Autodesk Inventor part; units mm, degrees
ref_plane "YZ Plane" through (0, 0, 0) normal (1, 0, 0) x (0, 1, 0)
ref_plane "XZ Plane" through (0, 0, 0) normal (0, 1, 0) x (-1, 0, 0)
ref_plane "XY Plane" through (0, 0, 0) normal (0, 0, 1) x (1, 0, 0)
sketch "Boceto1" plane through (0, 0, 0) normal (0, 1, 0) x (-1, 0, 0)
  line L0 (70.0475, 27.7623) -> (-31.8125, 27.7623)
  line L1 (-31.8125, 27.7623) -> (-31.8125, -25.8477)
  line L2 (-31.8125, -25.8477) -> (70.0475, -25.8477)
  line L3 (70.0475, -25.8477) -> (70.0475, 27.7623)
  point P0 (0, 0)
  dimension "d0" = 53.61
  dimension "d1" = 101.86
extrude "Extrusión1" add sketch "Boceto1" along normal blind 2
sketch "Boceto6" plane through (0, 0, 0) normal (0, -1, 0) x (1, 0, 0)
  line L0 (-50.0475, 27.7623) -> (23.8125, 27.7623)
  line L1 (28.8125, 27.7623) -> (31.8125, 24.7623)
  line L2 (31.8125, 27.7623) -> (31.8125, -25.8477)
  line L3 (-70.0475, 27.7623) -> (31.8125, 27.7623)
  line L4 (28.8125, 27.7623) -> (31.8125, 27.7623)
  line L5 (31.8125, 27.7623) -> (31.8125, 24.7623)
  circle A0 centre (25.3125, 25.7623) radius 1.5
  line L6 (31.8125, 17.7623) -> (31.8125, -25.8477)
  line L7 (31.8125, -15.8477) -> (25.8125, -25.8477)
  line L8 (31.8125, -25.8477) -> (23.8125, -25.8477)
  line L9 (31.8125, -25.8477) -> (28.8125, -25.8477)
  line L10 (28.8125, -25.8477) -> (28.8125, 5.0493)
  line L11 (28.8125, -10.8477) -> (31.8125, -5.8477)
  line L12 (31.8125, -5.8477) -> (31.8125, -25.8477)
  line L13 (25.8125, -25.8477) -> (31.8125, -25.8477)
  circle A1 centre (16.8125, -23.8477) radius 1.5
  line L14 (31.8125, -25.8477) -> (-70.0475, -25.8477)
  circle A2 centre (-56.0475, 25.7623) radius 1.5
  line L15 (-70.0475, 27.7623) -> (31.8125, 27.7623)
  line L16 (-70.0475, -25.8477) -> (-70.0475, 27.7623)
  circle A3 centre (-55.0475, -23.8477) radius 1.5
  point P0 (0, 0)
  point P1 (28.8125, -20.8477)
  point P2 (28.8125, -20.8477)
  dimension "d39" = 3
  dimension "d40" = 3
  dimension "d41" = 3
  dimension "d42" = 6.5
  dimension "d43" = 2
  dimension "d44" = 6
  dimension "d45" = 10
  dimension "d46" = 3
  dimension "d47" = 10
  dimension "d48" = 10
  dimension "d49" = 3
  dimension "d50" = 2
  dimension "d51" = 15
  dimension "d52" = 3
  dimension "d53" = 2
  dimension "d54" = 14
  dimension "d55" = 3
  dimension "d56" = 2
  dimension "d57" = 15
extrude "Extrusión7" cut sketch "Boceto6" against normal blind 3 contours L3 L2 L1 | L7 L10 L8 | L2 L7 L10 L11 | L7 L2 L8 L10 | A0 | A1 | A2 | A3
sketch "Boceto5" plane through (0, 2, 0) normal (0, 1, 0) x (1, 0, 0)
  line L0 (-73.0475, -22.7623) -> (-58.0475, -22.7623)
  line L1 (-58.0475, -22.7623) -> (-58.0475, -15.7623)
  line L2 (-58.0475, -15.7623) -> (-73.0475, -15.7623)
  line L3 (-73.0475, -15.7623) -> (-73.0475, -22.7623)
  line L4 (-70.0475, -27.7623) -> (31.8125, -27.7623)
  line L5 (-70.0475, 25.8477) -> (-70.0475, -27.7623)
  point P0 (0, 0)
  point P1 (-50.0475, -27.7623)
  point P2 (-65.5475, -22.7623)
  dimension "d33" = 5
  dimension "d34" = 7
  dimension "d35" = 3
  dimension "d36" = 15
extrude "Extrusión6" add sketch "Boceto5" along normal blind 8
sketch "Boceto4" plane through (0, 2, 0) normal (0, 1, 0) x (1, 0, 0)
  line L0 (-52.9032, 4.2581) -> (-20.9032, 4.2581)
  line L1 (-20.9032, 4.2581) -> (-20.9032, 9.2581)
  line L2 (-20.9032, 9.2581) -> (-52.9032, 9.2581)
  line L3 (-52.9032, 9.2581) -> (-52.9032, 4.2581)
  line L4 (-1.1875, -7.7419) -> (3.8125, -7.7419)
  line L5 (3.8125, -7.7419) -> (3.8125, 4.2581)
  line L6 (3.8125, 4.2581) -> (-1.1875, 4.2581)
  line L7 (-1.1875, 4.2581) -> (-1.1875, -7.7419)
  line L8 (23.8125, 25.8477) -> (23.8125, -17.7623)
  point P0 (0, 0)
  point P1 (-36.9032, 9.2581)
  point P2 (-36.9032, 4.2581)
  point P3 (1.3125, 4.2581)
  point P4 (1.3125, -7.7419)
  point P5 (-1.1875, -1.7419)
  point P6 (3.8125, -1.7419)
  point P7 (-20.9032, 6.7581)
  point P8 (-52.9032, 6.7581)
  dimension "d19" = 5
  dimension "d20" = 12
  dimension "d21" = 5
  dimension "d22" = 32
  dimension "d23" = 20
extrude "Extrusión4" add sketch "Boceto4" along normal blind 8
sketch "Boceto7" plane through (0, 2, 0) normal (0, 1, 0) x (1, 0, 0)
  line L0 (27.3125, 20.8477) -> (22.3125, 20.8477)
  line L1 (22.3125, 20.8477) -> (22.3125, -22.1523)
  line L2 (22.3125, -22.1523) -> (27.3125, -22.1523)
  line L3 (27.3125, -22.1523) -> (27.3125, 20.8477)
  line L4 (28.8125, 10.8477) -> (28.8125, 20.8477)
  line L5 (25.8125, 25.8477) -> (-70.0475, 25.8477)
  line L6 (21.8125, -23.2623) -> (-43.1875, -23.2623)
  line L7 (-43.1875, -23.2623) -> (-43.1875, -26.2623)
  line L8 (-43.1875, -26.2623) -> (21.8125, -26.2623)
  line L9 (21.8125, -26.2623) -> (21.8125, -23.2623)
  line L10 (-70.0475, -27.7623) -> (28.8125, -27.7623)
  line L11 (31.8125, -24.7623) -> (31.8125, 5.8477)
  line L12 (13.8125, 24.3477) -> (-52.0475, 24.3477)
  line L13 (-52.0475, 24.3477) -> (-52.0475, 21.3477)
  line L14 (-52.0475, 21.3477) -> (13.8125, 21.3477)
  line L15 (13.8125, 21.3477) -> (13.8125, 24.3477)
  line L16 (-70.0475, 25.8477) -> (-70.0475, -15.7623)
  point P0 (0, 0)
  point P1 (24.8125, 20.8477)
  point P2 (21.8125, -24.7623)
  point P3 (-43.1875, -24.7623)
  point P4 (13.8125, 22.8477)
  point P5 (-52.0475, 22.8477)
  dimension "d60" = 1.5
  dimension "d61" = 5
  dimension "d62" = 5
  dimension "d63" = 43
  dimension "d64" = 1.5
  dimension "d65" = 3
  dimension "d66" = 10
  dimension "d67" = 65
  dimension "d68" = 1.5
  dimension "d69" = 3
  dimension "d70" = 15
  dimension "d71" = 18
extrude "Extrusión8" add sketch "Boceto7" along normal blind 8
properties part number "Wemos Mega"
Here's how the part is built. I have some questions about the finished solid (model axes, mm). A direction names the side the tool comes from. Coordinates: 2 decimals unless noted, no trailing zeros. Loops run counter-clockwise (first coordinate to the right, second up) from the corner with the lowest first, then second, coordinate; pieces in that order, holes last. Notation, with made-up numbers: M 64.5,14.5 L 97.5,14.5 A17 cw 97.5,44.5 Z; hole C -8,89 d8. An arc over 180 degrees is marked long. One line per item, written item: value.
1. Thinking about a two-plate mould opening in X: for faces 5 (the flat face through (27.312, 6, 1)), 6 (the cylindrical face through (-56.24, 0.99, -24.76)), 7 (the flat face through (-70.048, 1, 1)), 8 (the flat face through (25, 10, 0)), which applies, +X half, -X half, draft (parallel to the pull), parting line (faces both ways), or undercut?
Geometry says:
face 5: +X half
face 6: undercut
face 7: -X half
face 8: draft
2. Imagine slicing it at A-A (y = 8). List the corners of the cut face in (x, z) for me, and give its area (3 significant figures).
Geometry says:
outline: M -73.05,15.76 L -58.05,15.76 L -58.05,22.76 L -73.05,22.76 Z; M -52.9,-9.26 L -20.9,-9.26 L -20.9,-4.26 L -52.9,-4.26 Z; M -52.05,-24.35 L 13.81,-24.35 L 13.81,-21.35 L -52.05,-21.35 Z; M -43.19,23.26 L 21.81,23.26 L 21.81,26.26 L -43.19,26.26 Z; M -1.19,-4.26 L 3.81,-4.26 L 3.81,7.74 L -1.19,7.74 Z; M 22.31,-20.85 L 27.31,-20.85 L 27.31,22.15 L 22.31,22.15 Z
area: 933 mm2
3. On a 3-axis mill with a long thin cutter (end or side, diameter ignored), from which of +Z, -Z, +X, -X, +Y, -Y can I reach the whole of each face in a straight line? I mean faces 1 (the flat face through (-72, 2, 19)), 2 (the flat face through (-11, 6, 26.262)), 3 (the flat face through (-43.188, 6, 25)), 4 (the flat face through (25, 6, 22.152)). Say none if no direction works.
Geometry says:
face 1: +Z, -Z, -X, -Y
face 2: +Z, +X, -X, +Y
face 3: +Z, -X, +Y
face 4: +Z, +X, +Y
4. Imagine slicing it at B-B (z = 18). List the corners of the cut face in (x, y) for me.
Geometry says:
outline: M -73.05,2 L -70.05,2 L -70.05,0 L 31.81,0 L 31.81,2 L 27.31,2 L 27.31,10 L 22.31,10 L 22.31,2 L -58.05,2 L -58.05,10 L -73.05,10 Z
5. Imagine slicing it at D-D (z = -15). List the corners of the cut face in (x, y) for me, and give its area (3 significant figures).
Geometry says:
outline: M -70.05,0 L 28.81,0 L 28.81,2 L 27.31,2 L 27.31,10 L 22.31,10 L 22.31,2 L -70.05,2 Z
area: 238 mm2
6. Please list where these lines run through material, in increasing order: probe 1 along Z at (x, y) = (-22, 9.25); probe 2 along Z at (x, y) = (3.5, 8.75); probe 3 along X at (y, z) = (7.25, -0.5).
Geometry says:
probe 1: z = -24.35 to -21.35, -9.26 to -4.26, 23.26 to 26.26
probe 2: z = -24.35 to -21.35, -4.26 to 7.74, 23.26 to 26.26
probe 3: x = -1.19 to 3.81, 22.31 to 27.31
7. Will these pins go through, and if not, where does the flat tip stop? pin 1 Ø3.5 at (y, z) = (7, 25) entering from +X; pin 2 Ø3.5 at (y, z) = (6.5, 19) entering from +X; pin 3 Ø3.5 at (x, z) = (-56.05, 25.76) entering from +Y.
Geometry says:
pin 1: stops at x = 21.81
pin 2: stops at x = 27.31
pin 3: stops at y = 2
8. Imagine slicing it at C-C (x = -46). List the corners of the cut face in (y, z) for me.
Geometry says:
outline: M 0,-25.85 L 2,-25.85 L 2,-24.35 L 10,-24.35 L 10,-21.35 L 2,-21.35 L 2,-9.26 L 10,-9.26 L 10,-4.26 L 2,-4.26 L 2,27.76 L 0,27.76 Z
